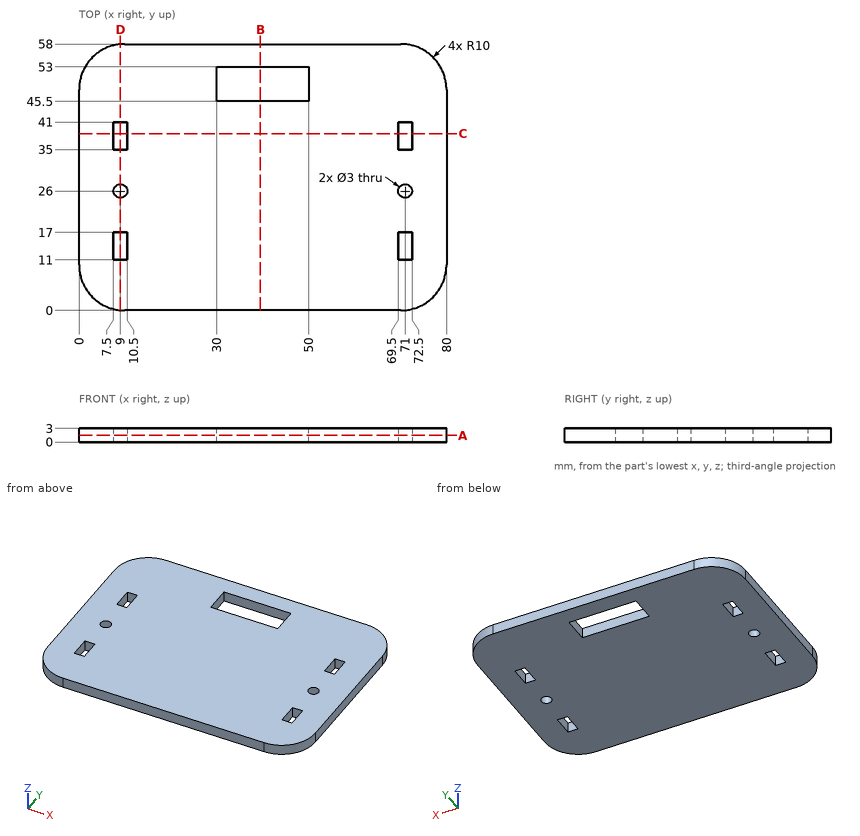
Here's the drawing with two shaded views (mm, measured from the low corner). I have some questions. Round coordinates to 2 decimals unless told otherwise and drop trailing zeros. Order: outer loops, then holes, each group sorted by start corner. A loop starts at its lowest first (then second) coordinate and runs counter-clockwise, first axis right, second up. Notation, with made-up numbers: M 82,9.25 L 115,9.25 A24 ccw 115,20.25 Z; hole C 74.25,-21.5 d4. An arc over 180 degrees is marked long. Use CSV: the item, a comma, the result in double quotes.
1) I want a section at B-B (x = 39.5). List the corners of the cut face in (y, z) for me, then the cut area to 4 significant figures.
Taken from the geometry:
outline,"M 0,0 L 45.5,0 L 45.5,3 L 0,3 Z; M 53,0 L 58,0 L 58,3 L 53,3 Z"
area,"151.5 mm^2"
2) I want a section at C-C (y = 38.5). List the corners of the cut face in (x, z) for me.
Taken from the geometry:
outline,"M 0,0 L 7.5,0 L 7.5,3 L 0,3 Z; M 10.5,0 L 69.5,0 L 69.5,3 L 10.5,3 Z; M 72.5,0 L 80,0 L 80,3 L 72.5,3 Z"
3) I'm going to push flat-ended pins straight in: P1, Ø1.5, axis at x = 9, z = 1.5, coming from the +Y side; P2, Ø0.9, axis at y = 49, z = 1.5, coming from the -X side. Where does each tip first touch, or does it pass through?
Taken from the geometry:
P1,"y = 58"
P2,"x = 0.02"
4) I want a section at A-A (z = 1.5). Count the separate pieces of the cut face and the enclosed holes in it, then the cut area to 3 significant figures.
Taken from the geometry:
separate pieces,"1"
enclosed holes,"7"
area,"4,320 mm^2"
5) I want a section at D-D (x = 9). List the corners of the cut face in (y, z) for me, then the cut area to 3 significant figures.
Taken from the geometry:
outline,"M 0.05,0 L 11,0 L 11,3 L 0.05,3 Z; M 17,0 L 24.5,0 L 24.5,3 L 17,3 Z; M 27.5,0 L 35,0 L 35,3 L 27.5,3 Z; M 41,0 L 57.95,0 L 57.95,3 L 41,3 Z"
area,"129 mm^2"
6) I need wall thicknesses on line 1 along X through (y, z) = (13, 0.5); line 2 along Y through (x, z) = (9, 2); line 3 along Y through (x, z) = (33, 2.2). Which ranges of each line are inside material? Lowest first, please. Write a range as [from, to].
Taken from the geometry:
line 1,"[0, 7.5], [10.5, 69.5], [72.5, 80]"
line 2,"[0.05, 11], [17, 24.5], [27.5, 35], [41, 57.95]"
line 3,"[0, 45.5], [53, 58]"
